Build history of the part. All positions in model axes, mm. A direction names the side the tool comes from. Give positions to 0.01 mm unless a question says otherwise; leave off trailing zeros. Order: outer loops, then holes, each group sorted by start corner. A loop starts at its lowest first (then second) coordinate and runs counter-clockwise, first axis right, second up. Notation, with made-up numbers: (-4.5, 31.5) - (36.5, 31.5) arc R16 ccw to (36.5, 38.5) - close; hole circle Ø6 at (72.5, 7.25). An arc over 180 degrees is marked (long way). Answer in a Markdown table with one row per item.
```python
from build123d import *

# Parameters (mm, degrees)
F1_DEPTH = 14
F2_R     = 1.35
F3_DEPTH = 17
F5_R     = 1
F6_DEPTH = 25


with BuildPart() as f1:
    # F0 (on Top) → F1 (new body)
    with BuildSketch(Plane.XY):
        Polygon((-20.125, 1.25), (-20.5, 0), (-22.5, 0), (-22.5, -1.25), (-20.5, -1.25), (5.125, -1.25), (5.125, 0), (2.55, 0), (2.175, 1.25), (0.375, 1.25), (0, 0), (-2.575, 0), (-2.95, 1.25), (-4.75, 1.25), (-5.125, 0), (-7.7, 0), (-8.075, 1.25), (-9.875, 1.25), (-10.25, 0), (-12.825, 0), (-13.2, 1.25), (-15, 1.25), (-15.375, 0), (-17.95, 0), (-18.325, 1.25), align=None)
    extrude(amount=F1_DEPTH)


with BuildPart() as f3:
    # F2 (on Top) → F3 (new body)
    with BuildSketch(Plane.XY):
        with BuildLine():
            Line((5.125, -3.25), (5.125, 3.25))
            Line((5.125, 3.25), (-6.6875, 3.25))
            ThreePointArc((-6.6875, 3.25), (-8.6875, 5.25), (-10.6875, 3.25))
            Line((-10.6875, 3.25), (-22.5, 3.25))
            Line((-22.5, 3.25), (-22.5, -3.25))
            Line((-22.5, -3.25), (5.125, -3.25))
        make_face()
        with Locations((-8.6875, 3.25)):
            Circle(F2_R, mode=Mode.SUBTRACT)
    extrude(amount=F3_DEPTH)

    # F4: cut F1
    add(f1.part, mode=Mode.SUBTRACT)

    # F5 (on face) → F6 (cut)
    with BuildSketch(Plane.XZ.offset(3.25)):
        with Locations((-13.6875, 5)):
            Circle(F5_R)
    extrude(amount=-F6_DEPTH, mode=Mode.SUBTRACT)


solid = f3.part
```
1. Two-plate mould, pull along Y, no slides. Class faces 1 (the face through (-8.64, 5.25, 8.38)), 2 (the face through (-4.935, 0.634, 6.902)), 3 (the face through (-12.734, -2.264, 5.3)): +Y half, -Y half, draft (parallel to the pull), parting line (faces both ways), or undercut.
Check result:
| item | result |
|---|---|
| face 1 | +Y half |
| face 2 | undercut |
| face 3 | draft |
2. Which spindle directions (+Z, -Z, +X, -X, +Y, -Y) get a long thin tool onto all of the face, cutting with end or side? Do faces 4 (the face through (-22.5, 1, 8)), 5 (the face through (-14, 1.25, 7)), 6 (the face through (-21, 0, 7)). Say none if no direction does.
Check result:
| item | result |
|---|---|
| face 4 | +Z, -Z, -X, +Y, -Y |
| face 5 | -Z |
| face 6 | -Z, +X, -X |
3. Probe line 1 (Y direction, x = -13.25, z = 8); line 2 (Y direction, x = -15.75, z = 2.75); line 3 (X direction, y = 1, z = 12) (3 decimals). List the from-to ranges inside material, lowest first.
Check result:
| item | result |
|---|---|
| line 1 | y = -3.25 to -1.25, 1.25 to 3.25 |
| line 2 | y = -3.25 to -1.25, 0 to 3.25 |
| line 3 | x = -22.5 to -20.2, -18.25 to -15.075, -13.125 to -9.95, -8 to -4.825, -2.875 to 0.3, 2.25 to 5.125 |
4. Drop flat-ended pins along their axis: P1, Ø2.5, axis at x = -13.69, z = 5, coming from the -Y side; P2, Ø7, axis at x = -3, z = 9.5, coming from the +Y side. Give the stop position or say it passes through.
Check result:
| item | result |
|---|---|
| P1 | stops at y = -3.25 |
| P2 | stops at y = 3.25 |
5. Cut at C-C on x = -9. Write the cut outline in (y, z).
Check result:
| item | result |
|---|---|
| outline | (-3.25, 0) - (-1.25, 0) - (-1.25, 14) - (1.25, 14) - (1.25, 0) - (1.94, 0) - (1.94, 17) - (-3.25, 17) - close; (4.56, 0) - (5.23, 0) - (5.23, 17) - (4.56, 17) - close |
6. Cut at A-A on z = 8.75. Count the separate pieces of the cut face and the enclosed holes in it, and give its area (3 significant figures).
Check result:
| item | result |
|---|---|
| separate pieces | 2 |
| enclosed holes | 1 |
| area | 132 mm² |
